Autodesk Inventor part; units mm, degrees
ref_plane "YZ Plane" through (0, 0, 0) normal (1, 0, 0) x (0, 1, 0)
ref_plane "XZ Plane" through (0, 0, 0) normal (0, 1, 0) x (-1, 0, 0)
ref_plane "XY Plane" through (0, 0, 0) normal (0, 0, 1) x (1, 0, 0)
sketch "Sketch1" plane through (0, 0, 0) normal (0, 0, 1) x (1, 0, 0)
  line L0 (-325.0867, -79.7187) -> (100.1146, -4.7443)
  arc A0 (100.1146, -4.7443) -> (197.2008, 110.9585) centre (79.7131, 110.9585) ccw
  line L1 (197.2008, 110.9585) -> (197.2008, 182.1453)
  line L2 (194.0258, 182.1453) -> (197.2008, 182.1453)
  line L3 (194.0258, 182.1453) -> (194.0258, 110.9585)
  arc A1 (99.5632, -1.6175) -> (194.0258, 110.9585) centre (79.7131, 110.9585) ccw
  line L4 (99.5632, -1.6175) -> (-325.0867, -76.4948)
  line L5 (-325.0867, -79.7187) -> (-325.0867, -76.4948)
  point P0 (0, 0)
extrude "Extrusion1" add sketch "Sketch1" along normal blind 117.475
hole "Hole1" at (197.2008, 169.4453, 109.5375) direction (-1, 0, 0) diameter 6.731 depth 25.4 tip angle 118
pattern_linear "Rectangular Pattern1" count 2 spacing 68.2625 along (0, 0, -1) of "Hole1"
hole "Hole2" at (-312.5797, -77.5134, 109.5375) direction (-0.1736482, 0.9848078, 0) diameter 6.731 depth 25.4 tip angle 118
pattern_linear "Rectangular Pattern2" count 2 spacing 68.2625 along (0, 0, -1) of "Hole2"
pattern_linear "Rectangular Pattern3" count 2 spacing 368.3 along (0.9848078, 0.1736482, 0) of "Hole2"
properties part number "GE-12087-02"
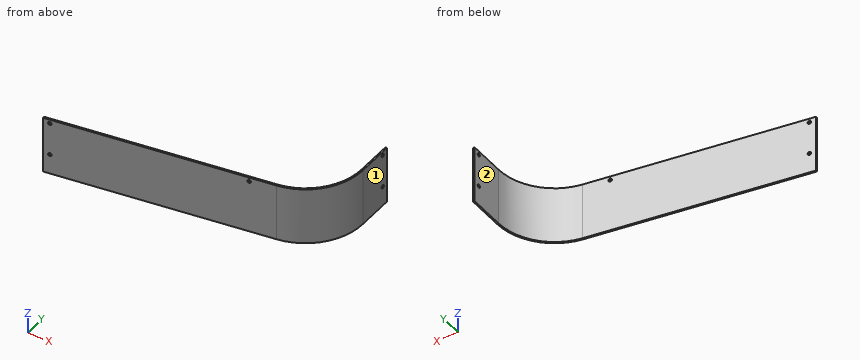
Build history of the part. All positions in model axes, mm. Face numbers are marked on the shaded views. A direction names the side the tool comes from. Round coordinates to 2 decimals unless told otherwise and drop trailing zeros. Loops run counter-clockwise (first coordinate to the right, second up) from the corner with the lowest first, then second, coordinate; pieces in that order, holes last. Notation, with made-up numbers: (-14.75, -8) -> (22.25, -8) arc R24 ccw to (22.25, 13) -> close; hole circle Ø1 at (88, 56). An arc over 180 degrees is marked (long way). Answer in a Markdown table with one row per item.
Item 1: Saw through at B-B (y = 122). Write the cut outline in (x, z) (3 decimals).
Answers below:
| item | result |
|---|---|
| outline | (194.026, 0) -> (197.201, 0) -> (197.201, 117.475) -> (194.026, 117.475) -> close |
Item 2: Drill centre lines: L1, parallel to X at y = 150, z = 50; L2, parallel to X at y = 29, z = 92; L3, parallel to Y at x = 113, z = 106. Where is each one in solid material? Low to high. Write a range as [from, to].
Answers below:
| item | result |
|---|---|
| L1 | x = [194.03, 197.2] |
| L2 | x = [159.4, 163.89] |
| L3 | y = [-1.72, 1.6] |
Item 3: Saw through at A-A (z = 75.5). Write the cut outline in (x, y).
Answers below:
| item | result |
|---|---|
| outline | (-325.09, -79.72) -> (100.11, -4.74) arc R117.49 ccw to (197.2, 110.96) -> (197.2, 182.15) -> (194.03, 182.15) -> (194.03, 110.96) arc R114.31 cw to (99.56, -1.62) -> (-325.09, -76.49) -> close |
Item 4: Which spindle directions (+Z, -Z, +X, -X, +Y, -Y) get a long thin tool onto all of the face, cutting with end or side? Do the marked faces 1 and 2. Say none if no direction does.
Answers below:
| item | result |
|---|---|
| face 1 | +Z, -Z, +X, +Y, -Y |
| face 2 | +Z, -Z, -X, +Y |
Item 5: Saw through at C-C (x = 62). Write the cut outline in (y, z) (3 decimals), and give its area (3 significant figures).
Answers below:
| item | result |
|---|---|
| outline | (-11.465, 0) -> (-8.241, 0) -> (-8.241, 117.475) -> (-11.465, 117.475) -> close |
| area | 379 mm² |
Item 6: Pin check, flat tips, straight feed: pin 1 (8 mm diameter, centred on x = -196.5, z = 37, fed in from +Y); pin 2 (4 mm diameter, centred on y = 169.45, z = 109.54, fed in from -X) (3 decimals); pin 3 (1.5 mm diameter, centred on y = 112, z = 58, fed in from -X); pin 4 (1.5 mm diameter, centred on x = -57.5, z = 23.5, fed in from -Y). Stop position of each tip, or through.
Answers below:
| item | result |
|---|---|
| pin 1 | stops at y = -53.12 |
| pin 2 | passes through |
| pin 3 | stops at x = 194.03 |
| pin 4 | stops at y = -32.67 |
